Work out the finished part from the listing and answer in its coordinate system (mm). Face numbers are marked on the shaded views. Round coordinates to 2 decimals unless told otherwise and drop trailing zeros.
Autodesk Inventor part; units mm, degrees
ref_plane "YZ Plane" through (0, 0, 0) normal (1, 0, 0) x (0, 1, 0)
ref_plane "XZ Plane" through (0, 0, 0) normal (0, 1, 0) x (-1, 0, 0)
ref_plane "XY Plane" through (0, 0, 0) normal (0, 0, 1) x (1, 0, 0)
sketch "Sketch1" plane through (0, 0, 0) normal (0, 1, 0) x (-1, 0, 0)
  line L0 (-10.5, 65.5) -> (-10.5, -65.5)
  line L1 (-10.5, 65.5) -> (-10.5, -65.5)
  line L2 (-10.5, -65.5) -> (-10.5, 65.5)
  line L3 (-10.5, -65.5) -> (-10.5, -30.5)
  line L4 (-10.5, 65.5) -> (-10.5, 30.15)
  line L5 (-10.5, 30.5) -> (-10.5, -30.5)
  line L6 (-10.5, 30.5) -> (-10.5, -30.5)
  circle A0 centre (-0.5, -30.5) radius 1.5
  line L7 (-10.5, -30.5) -> (-10.5, 30.15)
  circle A1 centre (-0.5, 30.15) radius 1.5
  line L8 (-10.5, -0.175) -> (20.5, -0.175)
  line L9 (-10.5, -0.175) -> (-10.5, -65.675)
  line L10 (-10.5, -0.175) -> (-10.5, 65.325)
  arc A2 (-10.5, 65.325) -> (-0.2045, 74.8119) centre (-7.9767, 72.9166) ccw
  arc A3 (-0.2045, -75.1619) -> (-10.5, -65.675) centre (-7.9767, -73.2666) ccw
  arc A4 (-0.2045, -75.1619) -> (-0.2045, 74.8119) centre (-125.6452, -0.175) ccw
  line L11 (-10.5, -65.675) -> (-10.5, 65.325)
  point P0 (0, 0)
  dimension "d13" = 35
  dimension "d14" = 35.35
  dimension "d17" = 3
  dimension "d21" = 3
  dimension "d24" = 31
  dimension "d27" = 65.5
  dimension "d28" = 65.5
  dimension "d35" = 14
  dimension "d36" = 8
  dimension "d37" = 14
  dimension "d38" = 8
extrude "Extrusion5" add sketch "Sketch1" along normal blind 13
fillet "Fillet1" radius 2 2 edges at (0.2045, 6.5, 74.8119) (0.2045, 6.5, -75.1619)
fillet "Fillet2" radius 2 12 edges at (-16.0052, 0, -36.1415) (-16.0052, 0, 35.7915) (-0.9895, 0, 70.5908) (4.8517, 0, 65.5522) (-0.9895, 0, -70.9408) (4.8517, 0, -65.9022) (-0.9895, 13, 70.5908) (4.8517, 13, 65.5522) (-0.9895, 13, -70.9408) (4.8517, 13, -65.9022) (-16.0052, 13, -36.1415) (-16.0052, 13, 35.7915)
properties part number "naraznik_kryt"
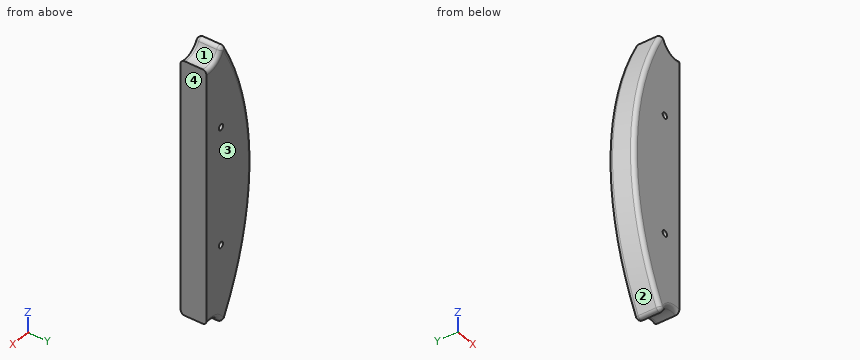
1. Find section A-A (y = 6.5). Give the number of separate pieces and of enclosed holes in the cut face, then the cut area to 3 significant figures.
Answer key:
separate pieces: 1
enclosed holes: 2
area: 3,440 mm2
2. Consider probe 1 along Z at (x, y) = (0.5, 5); probe 2 along X at (y, z) = (4, -30); probe 3 along Z at (x, y) = (-4.5, 12.25). Determine where each line is inside the solid, lowest interval first.
Answer key:
probe 1: z = -70.22 to -32, -29 to 28.65, 31.65 to 69.87
probe 2: x = -17.42 to -0.91, 1.91 to 10.5
probe 3: z = -65.7 to 65.35
3. Determine the mould class of the marked faces 1, 2, 3 and 4 for opening direction X: +X half, -X half, draft (parallel to the pull), parting line (faces both ways), or undercut.
Answer key:
face 1: undercut
face 2: -X half
face 3: draft
face 4: +X half
4. Given pin 1 (6 mm diameter, centred on x = 6.5, z = 53, fed in from -Y); pin 2 (3 mm diameter, centred on y = 4.5, z = -13.5, fed in from -X); pin 3 (1.5 mm diameter, centred on y = 6, z = 16.5, fed in from -X), each flat-ended and moving along its own axis, determine where each tip first touches the part or whether it passes through.
Answer key:
pin 1: stops at y = 0
pin 2: stops at x = -20.02
pin 3: stops at x = -19.63
